```python
from build123d import *

# Parameters (mm, degrees)
F0_W     = 70
F0_H     = 600
F1_DEPTH = 35
F2_R     = 12.7
F4_DEPTH = 72.39


with BuildPart() as f1:
    # F0 (on Front) → F1 (new body, symmetric)
    with BuildSketch(Plane.XZ):
        Rectangle(F0_W, F0_H)
    extrude(amount=F1_DEPTH, both=True)

    # F2
    f2_edges = [f1.edges().sort_by_distance(p)[0] for p in [
        (0, -35, 300),
        (0, 35, 300),
    ]]
    fillet(f2_edges, radius=F2_R)

    # F3 (on face) → F4 (cut, symmetric)
    with BuildSketch(Plane.XZ.offset(35)):
        Polygon((35, -300), (-35, -270), (-35, -300), align=None)
    extrude(amount=F4_DEPTH, both=True, mode=Mode.SUBTRACT)


solid = f1.part
```
The listing builds one solid part. Answer for the finished solid, in the listing's coordinates (mm). Coordinates: 2 decimals unless noted, no trailing zeros. Loops run counter-clockwise (first coordinate to the right, second up) from the corner with the lowest first, then second, coordinate; pieces in that order, holes last. Notation, with made-up numbers: M -23.5,83 L 17.5,83 A14 ccw 17.5,98 Z; hole C 87.5,9.25 d8. An arc over 180 degrees is marked long. Answer as a JSON object with one key per item and string values. Group by question number.
Item 1: Section A-A (x = -30) is taken. Write down the section's boundary in (y, z), and give its area (3 significant figures).
Item 2: Section C-C (x = 0.5) is taken. Write down the section's boundary in (y, z), and give its area (3 significant figures).
Item 3: This flat-tipped pin is pushed along its axis until it touches: P1, Ø1, axis at x = -24, y = 23, coming from the -Z side. Where does it stop, or does it pass through?
Item 4: Consider L1, parallel to Z at x = -18, y = 16.5; L2, parallel to Z at x = -9, y = -16.5; L3, parallel to X at y = 12, z = -275. Determine where each line is inside the solid, lowest interval first.
Item 5: Section B-B (y = -0.5) is taken. Write down the section's boundary in (x, z).
Solved:
{
 "1": {"outline": "M -35,-272.14 L 35,-272.14 L 35,287.3 A12.7 ccw 22.3,300 L -22.3,300 A12.7 ccw -35,287.3 Z", "area": "40,000 mm2"},
 "2": {"outline": "M -35,-285.21 L 35,-285.21 L 35,287.3 A12.7 ccw 22.3,300 L -22.3,300 A12.7 ccw -35,287.3 Z", "area": "40,900 mm2"},
 "3": {"P1": "stops at z = -274.93"},
 "4": {"L1": "z = -277.29 to 300", "L2": "z = -281.14 to 300", "L3": "x = -23.33 to 35"},
 "5": {"outline": "M -35,-270 L 35,-300 L 35,300 L -35,300 Z"}
}
